Check sheet for the modelled part. Datum: model origin and axes. Units: mm. Face numbers are marked on the shaded views. Round coordinates to 2 decimals unless told otherwise and drop trailing zeros.
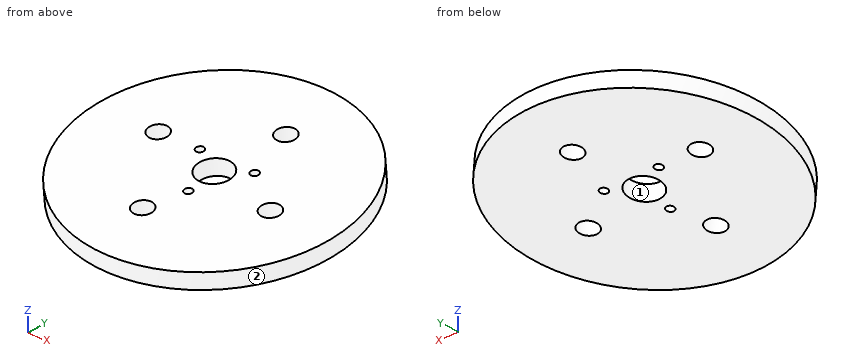
Autodesk Inventor part; units mm, degrees
ref_plane "Work Plane1" through (-85.339, 6.6926, 3.8884) normal (0.0215481, -0.1158759, 0.9930299) x (0.9954541, -0.0896829, -0.0320657)
ref_plane "YZ Plane" through (0, 0, 0) normal (1, 0, 0) x (0, 1, 0)
ref_plane "XZ Plane" through (0, 0, 0) normal (0, 1, 0) x (-1, 0, 0)
ref_plane "Work Plane1" through (-85.339, 6.6926, 3.8884) normal (0.0215481, -0.1158759, 0.9930299) x (0.9954541, -0.0896829, -0.0320657)
sketch "Sketch1" plane through (-85.339, 6.6926, 3.8884) normal (0.0215481, -0.1158759, 0.9930299) x (0.9954541, -0.0896829, -0.0320657)
  circle A0 centre (85.7068, 3.742) radius 3.175
  circle A1 centre (85.7068, 3.742) radius 24.765
  point P0 (85.676, 0.8558)
  dimension "d0" = 49.53
extrude "Extrusion1" add sketch "Sketch1" along normal blind 3.175
sketch "Sketch2" plane through (0.3253, 2.7078, 1.5645) normal (-0.0215481, 0.1158759, -0.9930299) x (-0.9997647, 0, 0.0216942)
  circle A0 centre (12.9454, 2.2936) radius 1.8542
  circle A1 centre (-2.2936, 12.9454) radius 1.8542
  circle A2 centre (-12.9454, -2.2936) radius 1.8542
  circle A3 centre (2.2936, -12.9454) radius 1.8542
extrude "Extrusion2" cut sketch "Sketch2" against normal through all
sketch "Sketch3" plane through (0.3937, 2.3399, 4.7174) normal (0.0215481, -0.1158759, 0.9930299) x (0.9997647, 0, -0.0216942)
  circle A0 centre (-5.246, 2.7309) radius 0.762
  circle A1 centre (4.988, 3.1777) radius 0.762
  circle A2 centre (0.258, -5.9086) radius 0.762
extrude "Extrusion3" cut sketch "Sketch3" against normal through all
properties part number "gearSpacerDisc01"
1. Release check for a two-part mould opening along X. For the marked faces 1 and 2 record: released by +X, released by -X, zero draft, split by the parting line, or undercut.
2. Scan lines: line 1 along Z through (x, y) = (-2, 5); line 2 along Z through (x, y) = (-10.5, 9); line 3 along X through (y, z) = (-16, 1.5). Record each from-to range of solid material in increasing order.
3. Go/stop test with flat-tipped pins: pin 1 (5 mm diameter, centred on y = -6.5, z = 1.5, fed in from -X); pin 2 (8 mm diameter, centred on x = -18.5, y = -5.5, fed in from +Z); pin 3 (3 mm diameter, centred on x = 17, z = 3.5, fed in from -Y). Record where each tip stops, or that it passes through.
Computed values:
1. face 1: undercut
1. face 2: split by the parting line
2. line 1: z = 1.88 to 5.08
2. line 2: z = 2.53 to 5.73
2. line 3: x = -16 to 16.74
3. pin 1: stops at x = -23.52
3. pin 2: stops at z = 4.69
3. pin 3: stops at y = -16.48
